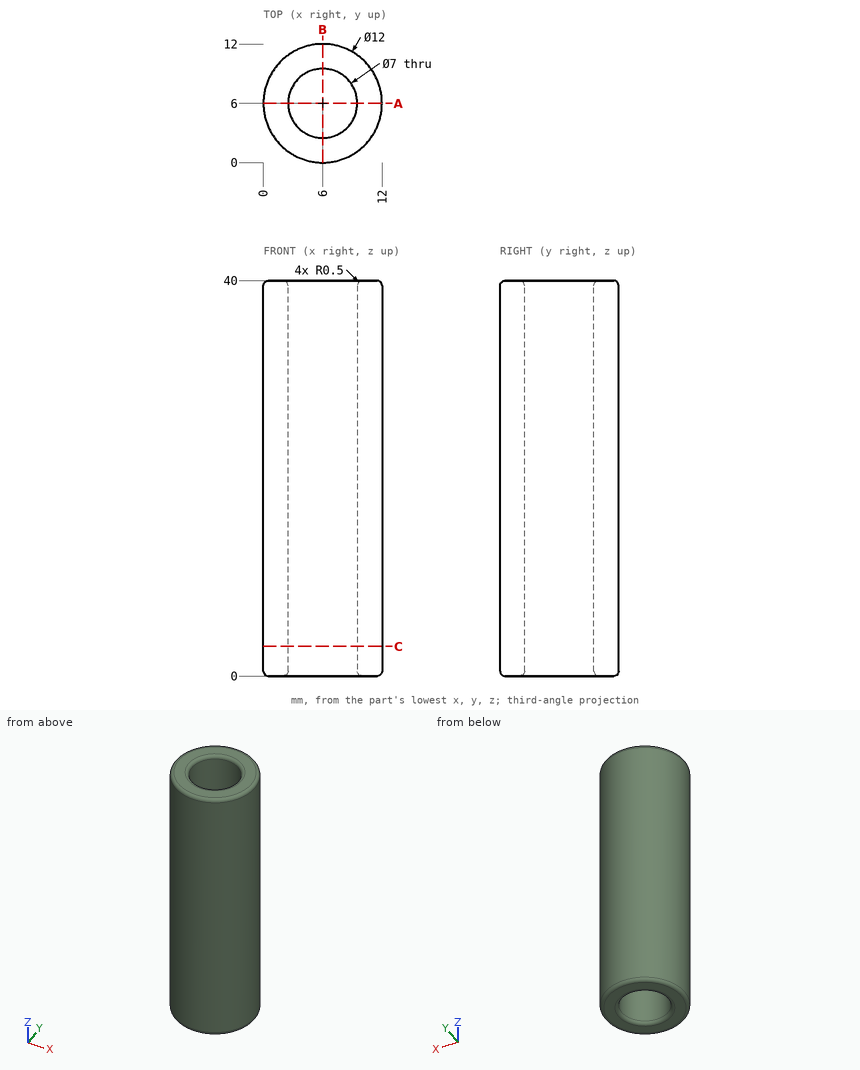
Source: three-view drawing plus pictorial views. Frame: mm from the lowest corner of the part. Round coordinates to 2 decimals unless told otherwise and drop trailing zeros. Loops run counter-clockwise (first coordinate to the right, second up) from the corner with the lowest first, then second, coordinate; pieces in that order, holes last.
Q1. Section A-A, the plane y = 6. Return loops of the section in (x, z).
Q2. Ray query, line 1 (Y direction, x = 6, z = 21); line 2 (X direction, y = 5.75, z = 37.5); line 3 (Y direction, x = 5, z = 14). Return the intervals inside material, ascending.
Q3. First-contact query: P1, Ø3, axis at x = 9, z = 20, coming from the +Y side; P2, Ø1.5, axis at y = 9, z = 21, coming from the +X side. Flat tips, straight axial feed; report the tip coordinate or a pass-through.
Q4. Section C-C, the plane z = 3. Return loops of the section in (x, y), plus the area to 3 significant figures.
Solutions:
1. outline: (0, 0.5) arc R0.5 ccw to (0.5, 0) - (2, 0) arc R0.5 ccw to (2.5, 0.5) - (2.5, 39.5) arc R0.5 ccw to (2, 40) - (0.5, 40) arc R0.5 ccw to (0, 39.5) - close; (9.5, 0.5) arc R0.5 ccw to (10, 0) - (11.5, 0) arc R0.5 ccw to (12, 0.5) - (12, 39.5) arc R0.5 ccw to (11.5, 40) - (10, 40) arc R0.5 ccw to (9.5, 39.5) - close
2. line 1: y = 0 to 2.5, 9.5 to 12
2. line 2: x = 0.01 to 2.51, 9.49 to 11.99
2. line 3: y = 0.08 to 2.65, 9.35 to 11.92
3. P1: stops at y = 11.81
3. P2: stops at x = 11.56
4. outline: circle Ø12 at (6, 6); hole circle Ø7 at (6, 6)
4. area: 74.6 mm2
